```python
from build123d import *
from build123d.topology import SkipClean

# Parameters (mm, degrees)
SKETCH_1_R          = 210
SKETCH_1_R_2        = 203
EXTRUDE_2_DEPTH     = 174
EXTRUDE_START       = -174
EXTRUDE_4_DEPTH     = 174
CUT_EXTRUDE_1_DEPTH = 654
EXTRUDE_5_DEPTH     = 174
EXTRUDE_6_DEPTH     = 174
EXTRUDE_7_DEPTH     = 174
EXTRUDE_8_DEPTH     = 174
CUT_EXTRUDE_START   = -654
CUT_EXTRUDE_2_DEPTH = 654
SKETCH_10_W         = 20.487801248
SKETCH_10_H         = 174
CUT_EXTRUDE_3_DEPTH = 327
SKETCH_11_W         = 235.63772895
SKETCH_11_H         = 249.192111589
CUT_EXTRUDE_4_DEPTH = 238
EXTRUDE_10_DEPTH    = 180
SKETCH_17_W         = 286.098661696
SKETCH_17_H         = 191.878669743
CUT_EXTRUDE_5_DEPTH = 322
EXTRUDE_11_DEPTH    = 180
SKETCH_20_R         = 4
CUT_EXTRUDE_7_DEPTH = 555.5
EXTRUDE_13_DEPTH    = 3
SKETCH_25_W         = 733.806449845
SKETCH_25_H         = 306.921913774
CUT_EXTRUDE_8_DEPTH = 240.5


with BuildPart() as part:
    # 草图1 → 凸台-拉伸2 (new body)
    with BuildSketch(Plane.XY):
        Circle(SKETCH_1_R)
        Circle(SKETCH_1_R_2, mode=Mode.SUBTRACT)
    extrude(amount=EXTRUDE_2_DEPTH)

    # 草图2 → 凸台-拉伸4 (add)
    with BuildSketch(Plane.XY.offset(174).offset(EXTRUDE_START)):
        with BuildLine():
            Line((-170.735431044, -102), (-173.735431044, -102))
            Line((-173.735431044, -102), (-175.513532242, -102))
            ThreePointArc((-175.513532242, -102), (-174.63092392, -103.50381834), (-173.735431044, -105))
            Line((-173.735431044, -105), (-170.735431044, -105))
            Line((-170.735431044, -105), (-170.735431044, -102))
        make_face()
        with BuildLine():
            ThreePointArc((173.735431044, -105), (174.63092392, -103.50381834), (175.513532242, -102))
            Line((175.513532242, -102), (173.735431044, -102))
            Line((173.735431044, -102), (170.735431044, -102))
            Line((170.735431044, -102), (170.735431044, -105))
            Line((170.735431044, -105), (173.735431044, -105))
        make_face()
    extrude(amount=EXTRUDE_4_DEPTH)

    # 草图3 → 切除-拉伸1 (cut)
    with BuildSketch(Plane.XY.offset(174)):
        Polygon((-170.735431044, -102), (238.333646515, -102), (254.334169784, 272.292523591), (-334.569415043, 221.85110305), (-306.830562533, -102), align=None)
    extrude(amount=-CUT_EXTRUDE_1_DEPTH, mode=Mode.SUBTRACT)

    # 草图5 → 凸台-拉伸5 (add)
    with BuildSketch(Plane.XY.offset(174).offset(EXTRUDE_START)):
        with BuildLine():
            Line((-120, -209.75), (-10.243900624, -209.75))
            ThreePointArc((-10.243900624, -209.75), (-67.755470707, -198.769203322), (-120, -172.336879396))
            Line((-120, -172.336879396), (-120, -209.75))
        make_face()
        with BuildLine():
            ThreePointArc((120, -172.336879396), (67.755470707, -198.769203322), (10.243900624, -209.75))
            Line((10.243900624, -209.75), (120, -209.75))
            Line((120, -209.75), (120, -172.336879396))
        make_face()
    extrude(amount=EXTRUDE_5_DEPTH)

    # 草图6 → 凸台-拉伸6 (add)
    with BuildSketch(Plane.XY.offset(174).offset(EXTRUDE_START)):
        with BuildLine():
            Line((-175.513532242, -102), (-166.195667814, -102))
            ThreePointArc((-166.195667814, -102), (0, -195), (166.195667814, -102))
            Line((166.195667814, -102), (175.513532242, -102))
            ThreePointArc((175.513532242, -102), (0, -203), (-175.513532242, -102))
        make_face()
    extrude(amount=EXTRUDE_6_DEPTH)

    # 草图7 → 凸台-拉伸7 (add)
    with BuildSketch(Plane.XY.offset(174).offset(EXTRUDE_START)):
        with BuildLine():
            Line((-166.933126535, -92), (-166.933126535, -95))
            Line((-166.933126535, -95), (-170.293863659, -95))
            ThreePointArc((-170.293863659, -95), (0, -195), (170.293863659, -95))
            Line((170.293863659, -95), (166.933126535, -95))
            Line((166.933126535, -95), (166.933126535, -92))
            Line((166.933126535, -92), (171.933126535, -92))
            Line((171.933126535, -92), (188.496850106, -92))
            ThreePointArc((188.496850106, -92), (0, -209.75), (-188.496850106, -92))
            Line((-188.496850106, -92), (-171.933126535, -92))
            Line((-171.933126535, -92), (-166.933126535, -92))
        make_face()
    extrude(amount=EXTRUDE_7_DEPTH)

    # 草图8 → 凸台-拉伸8 (add)
    with BuildSketch(Plane(origin=(0, 0, 0), x_dir=(-1, 0, 0), z_dir=(0, 0, -1))):
        with BuildLine():
            Line((166.933126535, -92), (163.933126535, -92))
            Line((163.933126535, -92), (163.933126535, -99))
            Line((163.933126535, -99), (168, -99))
            ThreePointArc((168, -99), (169.158755456, -97.006780447), (170.293863659, -95))
            Line((170.293863659, -95), (166.933126535, -95))
            Line((166.933126535, -95), (166.933126535, -92))
        make_face()
        with BuildLine():
            Line((-166.933126535, -95), (-170.293863659, -95))
            ThreePointArc((-170.293863659, -95), (-169.158755456, -97.006780447), (-168, -99))
            Line((-168, -99), (-163.933126535, -99))
            Line((-163.933126535, -99), (-163.933126535, -92))
            Line((-163.933126535, -92), (-166.933126535, -92))
            Line((-166.933126535, -92), (-166.933126535, -95))
        make_face()
    extrude(amount=-EXTRUDE_8_DEPTH)

    # 草图9 → 切除-拉伸2 (cut)
    with BuildSketch(Plane.XY.offset(174).offset(CUT_EXTRUDE_START)):
        with BuildLine():
            Line((0, -195), (0, -182.225251044))
            Line((0, -182.225251044), (-50, -182.225251044))
            Line((-50, -182.225251044), (-50, -188.48076825))
            ThreePointArc((-50, -188.48076825), (-25.211606368, -193.363323576), (0, -195))
        make_face()
        with BuildLine():
            Line((0, -209.75), (0, -195))
            ThreePointArc((0, -195), (-25.211606368, -193.363323576), (-50, -188.48076825))
            Line((-50, -188.48076825), (-50, -195))
            Line((-50, -195), (-50, -209.75))
            Line((-50, -209.75), (-10.243900624, -209.75))
            Line((-10.243900624, -209.75), (0, -209.75))
        make_face()
        with BuildLine():
            ThreePointArc((50, -188.48076825), (25.211606368, -193.363323576), (0, -195))
            Line((0, -195), (0, -209.75))
            Line((0, -209.75), (10.243900624, -209.75))
            Line((10.243900624, -209.75), (50, -209.75))
            Line((50, -209.75), (50, -195))
            Line((50, -195), (50, -188.48076825))
        make_face()
        with BuildLine():
            Line((50, -182.225251044), (0, -182.225251044))
            Line((0, -182.225251044), (0, -195))
            ThreePointArc((0, -195), (25.211606368, -193.363323576), (50, -188.48076825))
            Line((50, -188.48076825), (50, -182.225251044))
        make_face()
    extrude(amount=CUT_EXTRUDE_2_DEPTH, mode=Mode.SUBTRACT)


with BuildPart() as cut_extrude_2_piece_1:
    # of the separate pieces the step leaves, piece 1, a body of its own (cut_extrude_2_pieces)
    add(part.part.solids().sort_by_distance((-183.564702489, -102, 0))[0])

    # 草图11 → 切除-拉伸4 (cut)
    with BuildSketch(Plane(origin=(0, 0, 0), x_dir=(-1, 0, 0), z_dir=(0, 0, -1))):
        with Locations((136.586471206, -141.23053543)):
            Rectangle(SKETCH_11_W, SKETCH_11_H)
    extrude(amount=-CUT_EXTRUDE_4_DEPTH, mode=Mode.SUBTRACT)


with BuildPart() as cut_extrude_2_piece_2:
    # of the separate pieces the step leaves, piece 2, a body of its own (cut_extrude_2_pieces)
    add(part.part.solids().sort_by_distance((50, -188.48076825, 0))[0])

    # 草图17 → 切除-拉伸5 (cut)
    with BuildSketch(Plane(origin=(0, -92, 0), x_dir=(1, 0, 0), z_dir=(0, 1, 0))):
        with Locations((123.864076708, -90.777636372)):
            Rectangle(SKETCH_17_W, SKETCH_17_H)
    extrude(amount=-CUT_EXTRUDE_5_DEPTH, mode=Mode.SUBTRACT)


with BuildPart() as cut_extrude_2_piece_3:
    # of the separate pieces the step leaves, piece 3, a body of its own (cut_extrude_2_pieces)
    add(part.part.solids().sort_by_distance((10.243900624, -209.75, 0))[0])

    # 草图10 → 切除-拉伸3 (cut, symmetric)
    with BuildSketch(Plane(origin=(0, -209.75, 0), x_dir=(1, 0, 0), z_dir=(0, 1, 0))):
        with Locations((0, -87)):
            Rectangle(SKETCH_10_W, SKETCH_10_H)
    extrude(amount=CUT_EXTRUDE_3_DEPTH, both=True, mode=Mode.SUBTRACT)


with BuildPart() as body_2:
    # 草图14 → 凸台-拉伸10 (new body)
    with BuildSketch(Plane.XY.offset(209.75)):
        with BuildLine():
            Line((0, 210), (0, 205))
            ThreePointArc((0, 205), (174.477792283, 107.622023768), (183.196615689, -92))
            Line((183.196615689, -92), (188.774998345, -92))
            ThreePointArc((188.774998345, -92), (178.073018731, 111.310376875), (0, 210))
        make_face()
    extrude(amount=EXTRUDE_10_DEPTH)

    # 草图18 → 凸台-拉伸11 (add)
    with SkipClean():  # the faces are left unmerged after this step: merging them gives an invalid solid
        with BuildSketch(Plane.XY.offset(389.75)):
            with BuildLine():
                ThreePointArc((0, 210), (-178.073018731, 111.310376875), (-188.774998345, -92))
                Line((-188.774998345, -92), (-183.196615689, -92))
                ThreePointArc((-183.196615689, -92), (-174.477792283, 107.622023768), (0, 205))
                Line((0, 205), (0, 210))
            make_face()
        extrude(amount=-EXTRUDE_11_DEPTH)

    # 草图20 → 切除-拉伸7 (cut, symmetric)
    with SkipClean():  # the faces are left unmerged after this step: merging them gives an invalid solid
        with BuildSketch(Plane(origin=(0, 0, 0), x_dir=(0, 0, -1), z_dir=(1, 0, 0))):
            with Locations((-382.75, 98)):
                Circle(SKETCH_20_R)
        extrude(amount=CUT_EXTRUDE_7_DEPTH, both=True, mode=Mode.SUBTRACT)

    # 草图25 → 切除-拉伸8 (cut, symmetric)
    with BuildSketch(Plane(origin=(0, 0, 0), x_dir=(1, 0, 0), z_dir=(0, 1, 0))):
        with Locations((28.762967919, -312.90839884)):
            Rectangle(SKETCH_25_W, SKETCH_25_H)
    extrude(amount=CUT_EXTRUDE_8_DEPTH, both=True, mode=Mode.SUBTRACT)


with BuildPart() as body_2_2:
    # 草图24 → 凸台-拉伸13 (new body)
    with BuildSketch(Plane.XY):
        with BuildLine():
            Line((-184.187404564, 90), (0, 90))
            Line((0, 90), (184.187404564, 90))
            ThreePointArc((184.187404564, 90), (181.243442773, 95.790471613), (178.117498021, 101.484761905))
            ThreePointArc((178.117498021, 101.484761905), (0, 205), (-178.117498021, 101.484761905))
            ThreePointArc((-178.117498021, 101.484761905), (-181.243442773, 95.790471613), (-184.187404564, 90))
        make_face()
    extrude(amount=EXTRUDE_13_DEPTH)


solid = body_2_2.part
```
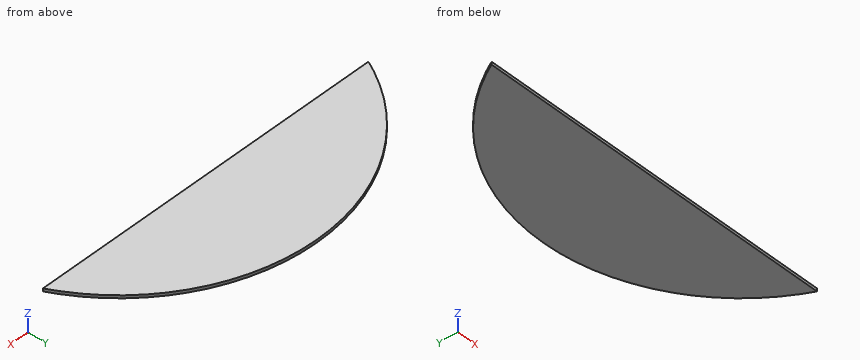
Source: CAD feature listing. Evaluate the final solid. Frame: model axes, mm. Round coordinates to 2 decimals unless told otherwise and drop trailing zeros. Loops run counter-clockwise (first coordinate to the right, second up) from the corner with the lowest first, then second, coordinate; pieces in that order, holes last. Notation, with made-up numbers: M 19,55 L 30,55 A15 ccw 30,81 Z; hole C -39.75,86 d2. An arc over 180 degrees is marked long. Use a Markdown table: item, result. Add a question column.
1. Section query B-B on y = 167.5. Return the cut outline in (x, z), then the cut area to 3 significant figures.
2. Section query A-A on z = 0.85. Return the cut outline in (x, y), then the cut area to 3 significant figures.
3. Line query: line 1 (X direction, y = 101.5, z = 2.45); line 2 (Y direction, x = -117.5, z = 2.4); line 3 (Y direction, x = -137.5, z = 0.15). Output: solid intervals per line, ascending.
Reported:
| question | item | result |
|---|---|---|
| 1 | outline | M -118.19,0 L 118.19,0 L 118.19,3 L -118.19,3 Z |
| 1 | area | 709 mm² |
| 2 | outline | M -184.19,90 L 184.19,90 A205 ccw Z |
| 2 | area | 30,300 mm² |
| 3 | line 1 | x = -178.11 to 178.11 |
| 3 | line 2 | y = 90 to 167.98 |
| 3 | line 3 | y = 90 to 152.05 |
